Verification items for the finished model (mm, model axes). A direction names the side the tool comes from. Coordinates: 2 decimals unless noted, no trailing zeros. Write each loop counter-clockwise with the first axis right and the second up, starting at its lowest first coordinate (ties: lowest second). Pieces come first, ordered by that corner, then holes. Notation, with made-up numbers: M 54,11.25 L 75,11.25 A12 cw 75,15.25 Z; hole C 53,2 d3. An arc over 180 degrees is marked long. One line per item, written item: value.
Autodesk Inventor part; units mm, degrees
ref_plane "YZ Plane" through (0, 0, 0) normal (1, 0, 0) x (0, 1, 0)
ref_plane "XZ Plane" through (0, 0, 0) normal (0, 1, 0) x (-1, 0, 0)
ref_plane "XY Plane" through (0, 0, 0) normal (0, 0, 1) x (1, 0, 0)
sketch "Sketch1" plane through (0, 0, 0) normal (0, 1, 0) x (-1, 0, 0)
  line L0 (45, 45) -> (-45, 45)
  line L1 (-45, 45) -> (-45, -45)
  line L2 (-45, -45) -> (45, -45)
  line L3 (45, -45) -> (45, 45)
  line L4 (45, 45) -> (-45, -45) construction
  line L5 (-45, 45) -> (45, -45) construction
  line L6 (-46, 46) -> (46, 46)
  line L7 (46, 46) -> (46, -46)
  line L8 (46, -46) -> (-46, -46)
  line L9 (-46, -46) -> (-46, 46)
  line L10 (-46, 46) -> (46, -46) construction
  line L11 (46, 46) -> (-46, -46) construction
  point P0 (0, 0)
  dimension "d0" = 90
  dimension "d1" = 90
  dimension "d2" = 92
  dimension "d3" = 92
extrude "Extrusion1" add sketch "Sketch1" along normal blind 1 contours L3 L2 L1 L0 | L6 L7 L8 L9
sketch "Sketch2" plane through (0, 1, 0) normal (0, 1, 0) x (1, 0, 0)
  line L0 (-46, -46) -> (46, -46)
  line L1 (46, -46) -> (46, 46)
  line L2 (46, 46) -> (-46, 46)
  line L3 (-46, 46) -> (-46, -46)
  line L4 (45, 45) -> (-45, 45)
  line L5 (-45, -20.5) -> (-45, -45)
  line L6 (-45, -45) -> (-17.75, -45)
  line L7 (45, -45) -> (45, 45)
  line L8 (45, 45) -> (-45, -45) construction
  line L9 (-45, 45) -> (45, -45) construction
  line L10 (-27.75, -30.5) -> (-17.75, -30.5)
  line L11 (-17.75, -30.5) -> (-17.75, -29.5)
  line L12 (-17.75, -29.5) -> (-27.75, -29.5)
  line L13 (-27.75, -29.5) -> (-27.75, -30.5)
  line L14 (-27.75, -30.5) -> (-26.75, -30.5)
  line L15 (-26.75, -30.5) -> (-26.75, -20.5)
  line L16 (-26.75, -20.5) -> (-27.75, -20.5)
  line L17 (-27.75, -20.5) -> (-27.75, -30.5)
  line L18 (-17.75, -45) -> (-17.75, -46)
  line L19 (-46, -46) -> (46, -46)
  line L20 (-45, -20.5) -> (-46, -20.5)
  point P0 (0, 0)
  dimension "d6" = 90
  dimension "d7" = 90
  dimension "d8" = 1
  dimension "d9" = 1
  dimension "d10" = 10
  dimension "d11" = 10
  dimension "d12" = 14.5
  dimension "d13" = 17.25
sketch "Sketch3" plane through (0, 1, 0) normal (0, 1, 0) x (1, 0, 0)
  line L0 (-27.75, -30.5) -> (-17.75, -30.5)
  line L1 (-27.75, -20.5) -> (-27.75, -30.5)
  line L2 (-26.75, -30.5) -> (-26.75, -20.5)
  line L3 (-17.75, -29.5) -> (-27.75, -29.5)
  line L4 (-26.75, -20.5) -> (-27.75, -20.5)
  line L5 (-17.75, -45) -> (-17.75, -46)
  line L6 (-45, -20.5) -> (-46, -20.5)
  line L7 (-46, 46) -> (-46, -46)
  line L8 (-45, -20.5) -> (-46, -20.5)
  line L9 (-46, -20.5) -> (-46, -46)
  line L10 (-46, -46) -> (-45, -46)
  line L11 (-45, -46) -> (-45, -20.5)
  line L12 (-46, -46) -> (46, -46)
  line L13 (-46, -46) -> (-17.75, -46)
  line L14 (-17.75, -46) -> (-17.75, -45)
  line L15 (-17.75, -45) -> (-46, -45)
  line L16 (-46, -45) -> (-46, -46)
  line L17 (-27.75, -30.5) -> (-17.75, -30.5)
  line L18 (-17.75, -30.5) -> (-17.75, -29.5)
  line L19 (-17.75, -29.5) -> (-27.75, -29.5)
  line L20 (-27.75, -29.5) -> (-27.75, -30.5)
  point P0 (0, 0)
extrude "Extrusion2" add sketch "Sketch3" along normal blind 7
sketch "Sketch4" plane through (-45, 1, 20.5) normal (0, 0, -1) x (-1, 0, 0)
  line L0 (-17.25, 0) -> (-18.25, 0)
  line L1 (-17.25, 0) -> (-17.25, 7)
  line L2 (-18.25, 7) -> (-17.25, 7)
  line L3 (-18.25, 0) -> (-18.25, 7)
  line L4 (1, 0) -> (0, 0)
  line L5 (1, 0) -> (1, 7)
  line L6 (0, 7) -> (1, 7)
  line L7 (0, 0) -> (0, 7)
  line L8 (0, 0) -> (-27.25, 0)
  arc A0 (-17.25, 4.027) -> (0, 4.027) centre (-8.625, 11.25) ccw
  line L9 (-91, 0) -> (1, 0)
  line L10 (-17.25, 0) -> (-17.25, 7)
  line L11 (-8.625, 0) -> (-17.25, 0)
  line L12 (-17.25, 0) -> (-17.25, 4.027)
  line L13 (0, 0) -> (0, 7)
  line L14 (-8.625, 0) -> (0, 0)
  line L15 (0, 0) -> (0, 4.027)
  point P0 (-45, -1)
  dimension "d16" = 22.5
  dimension "d17" = 8.625
extrude "Extrusion3" add sketch "Sketch4" against normal blind 10 contours A0 L7 L8 | L1 A0 L8
sketch "Sketch5" plane through (0, 1, 0) normal (0, 1, 0) x (1, 0, 0)
  line L0 (-17.75, -46) -> (46, -46)
  line L1 (-46, -20.5) -> (-46, -46)
  point P0 (0, 0)
  point P1 (-19, -19)
  dimension "d23" = 27
  dimension "d24" = 27
hole "Hole1" at (-19, 1, 19) direction (0, -1, 0) diameter 4 end through all
pattern_circular "Circular Pattern2" count 4 over 360 about axis through (0, -10, 0) along (0, 1, 0) of "Extrusion2", "Extrusion3", "Hole1"
sketch "Sketch6" plane through (0, 1, 0) normal (0, 1, 0) x (1, 0, 0)
  circle A0 centre (0, 0) radius 21
  dimension "d35" = 42
extrude "Extrusion4" cut sketch "Sketch6" against normal blind 10
sketch "Sketch7" plane through (0, 1, 0) normal (0, 1, 0) x (1, 0, 0)
  line L0 (45, 45) -> (-45, 45)
  line L1 (-45, 45) -> (-45, -45)
  line L2 (-45, -45) -> (45, -45)
  line L3 (45, -45) -> (45, 45)
  line L4 (45, 45) -> (-45, -45) construction
  line L5 (-45, 45) -> (45, -45) construction
  line L6 (46, -46) -> (-46, -46)
  line L7 (-46, 46) -> (46, 46)
  line L8 (46, 46) -> (46, -46)
  line L9 (46, -46) -> (-46, -46)
  line L10 (-46, -46) -> (-46, 46)
  line L11 (-46, 46) -> (46, -46) construction
  line L12 (46, 46) -> (-46, -46) construction
  point P0 (0, 0)
  dimension "d38" = 90
  dimension "d39" = 90
extrude "Extrusion5" add sketch "Sketch7" along normal blind 3
sketch "Sketch8" plane through (0, 1, 0) normal (0, 1, 0) x (1, 0, 0)
  circle A0 centre (-19, -19) radius 2
  circle A1 centre (19, -19) radius 2
  circle A2 centre (19, 19) radius 2
  circle A3 centre (-19, 19) radius 2
  circle A4 centre (0, 0) radius 21
  line L0 (-45, -45) -> (20.5, -45)
  line L1 (20.5, -45) -> (20.5, -36.375)
  line L2 (20.5, -36.375) -> (20.5, -26.75)
  line L3 (20.5, -26.75) -> (29.5, -26.75)
  line L4 (29.5, -26.75) -> (29.5, -17.75)
  line L5 (29.5, -17.75) -> (30.5, -17.75)
  line L6 (30.5, -17.75) -> (30.5, -36.375)
  line L7 (30.5, -36.375) -> (30.5, -45)
  line L8 (30.5, -45) -> (45, -45)
  line L9 (45, -45) -> (45, 20.5)
  line L10 (45, 20.5) -> (36.375, 20.5)
  line L11 (36.375, 20.5) -> (26.75, 20.5)
  line L12 (26.75, 20.5) -> (26.75, 29.5)
  line L13 (26.75, 29.5) -> (17.75, 29.5)
  line L14 (17.75, 29.5) -> (17.75, 30.5)
  line L15 (17.75, 30.5) -> (36.375, 30.5)
  line L16 (36.375, 30.5) -> (45, 30.5)
  line L17 (45, 30.5) -> (45, 45)
  line L18 (45, 45) -> (-20.5, 45)
  line L19 (-20.5, 45) -> (-20.5, 36.375)
  line L20 (-20.5, 36.375) -> (-20.5, 26.75)
  line L21 (-20.5, 26.75) -> (-29.5, 26.75)
  line L22 (-29.5, 26.75) -> (-29.5, 17.75)
  line L23 (-29.5, 17.75) -> (-30.5, 17.75)
  line L24 (-30.5, 17.75) -> (-30.5, 36.375)
  line L25 (-30.5, 36.375) -> (-30.5, 45)
  line L26 (-30.5, 45) -> (-45, 45)
  line L27 (-45, 45) -> (-45, -20.5)
  line L28 (-45, -20.5) -> (-36.375, -20.5)
  line L29 (-36.375, -20.5) -> (-26.75, -20.5)
  line L30 (-26.75, -20.5) -> (-26.75, -29.5)
  line L31 (-26.75, -29.5) -> (-17.75, -29.5)
  line L32 (-17.75, -29.5) -> (-17.75, -30.5)
  line L33 (-17.75, -30.5) -> (-36.375, -30.5)
  line L34 (-36.375, -30.5) -> (-45, -30.5)
  line L35 (-45, -30.5) -> (-45, -45)
  circle A5 centre (-19, -19) radius 2
  circle A6 centre (-19, -19) radius 4
  dimension "d42" = 8
extrude "Extrusion6" add sketch "Sketch8" along normal blind 10 contours A6
sketch "Sketch9" plane through (0, 0, 0) normal (0, -1, 0) x (1, 0, 0)
  circle A0 centre (0, 0) radius 21
  circle A1 centre (-19, -19) radius 2
  circle A2 centre (19, -19) radius 2
  circle A3 centre (19, 19) radius 2
  circle A4 centre (-19, 19) radius 2
  line L0 (46, 46) -> (-46, 46)
  line L1 (-46, 46) -> (-46, -46)
  line L2 (-46, -46) -> (46, -46)
  line L3 (46, -46) -> (46, 46)
  circle A5 centre (-19, 19) radius 3
  dimension "d45" = 6
extrude "Extrusion7" cut sketch "Sketch9" against normal blind 10 contours A5
fillet "Fillet1" radius 2 1 edges at (-23, 1, 19)
pattern_circular "Circular Pattern3" count 4 over 360 about axis through (0, -10, 0) along (0, 1, 0) of "Extrusion6", "Extrusion7", "Fillet1"
properties part number "motor_mount_base2_template"
Item 1: Go/stop test with flat-tipped pins: P1, Ø13, axis at x = 27.5, z = 33.5, coming from the +Y side; P2, Ø5, axis at x = 25, z = 23, coming from the +Y side; P3, Ø4, axis at x = -20, z = 10.5, coming from the +Y side; P4, Ø1.5, axis at y = 6.5, z = 5, coming from the -X side. Record where each tip stops, or that it passes through.
The answers:
P1: stops at y = 8
P2: stops at y = 1.47
P3: stops at y = 1
P4: passes through
Item 2: Draft check along X on faces 4 (the face through (27.75, 6, -25)), 5 (the face through (45.5, 8, 38.2)). Enter one of: released by +X, released by -X, zero draft, split by the parting line, or undercut.
The answers:
face 4: undercut
face 5: zero draft
Item 3: Cross-section at A-A, the plane z = 0. Enter the section's corners in (x, y), and give its area (3 significant figures).
The answers:
outline: M -46,0 L -21,0 L -21,1 L -45,1 L -45,4 L -46,4 Z; M 21,0 L 46,0 L 46,4 L 45,4 L 45,1 L 21,1 Z
area: 56.0 mm²
Item 4: Cross-section at C-C, the plane x = 19. Give the number of separate pieces and of enclosed holes in the cut face, and give its area (3 significant figures).
The answers:
separate pieces: 4
enclosed holes: 0
area: 127 mm²
Item 5: Access from +Z, -Z, +X, -X, +Y, -Y to the whole of each face (thin tool, end or side, straight path). Record for faces 1 (the face through (-19.26, 10.493, 20.983)), 2 (the face through (18, 10, -17)), 3 (the face through (29, 3, -20.5)).
The answers:
face 1: +Y, -Y
face 2: -Y
face 3: +Y
Item 6: Scan lines: line 1 (Z direction, x = -19, y = 10.65); line 2 (X direction, y = 5.5, z = -29); line 3 (Z direction, x = 34.5, y = 7.75). Record each from-to range of solid material in increasing order.
The answers:
line 1: z = -23 to -21, -17 to -15, 15 to 17, 21 to 23
line 2: x = -46 to -45, 26.75 to 27.75, 45 to 46
line 3: z = -46 to -45, 45 to 46
Item 7: Cross-section at B-B, the plane x = 0. Enter the section's corners in (y, z).
The answers:
outline: M 0,-46 L 4,-46 L 4,-45 L 1,-45 L 1,-21 L 0,-21 Z; M 0,21 L 1,21 L 1,45 L 4,45 L 4,46 L 0,46 Z
Item 8: Cross-section at D-D, the plane z = 39. Enter the section's corners in (x, y).
The answers:
outline: M -46,0 L 46,0 L 46,8 L 45,8 L 45,1 L 30.5,1 L 30.5,1.31 L 20.5,1.31 L 20.5,1 L -45,1 L -45,8 L -46,8 Z
